from build123d import *

# Parameters (mm, degrees)
CYLINDER003_R               = 0.62
CYLINDER003_DEPTH           = 0.5
CYLINDER002_R               = 0.62
CYLINDER002_DEPTH           = 0.5
CYLINDER001_R               = 0.62
CYLINDER001_DEPTH           = 0.5
CYLINDER001_PLACEMENT_ANGLE = -2
CYLINDER_R                  = 80
CYLINDER_DEPTH              = 0.5


with BuildPart() as cilindro003:
    # Cylinder003 → Cylinder003 (new body)
    with BuildSketch(Plane(origin=(0, 72, 0), x_dir=(1, 0, 0), z_dir=(0, 0, 1))):
        Circle(CYLINDER003_R)
    extrude(amount=CYLINDER003_DEPTH)


with BuildPart() as cilindro002:
    # Cylinder002 → Cylinder002 (new body)
    with BuildSketch(Plane(origin=(-72, -7, 0), x_dir=(1, 0, 0), z_dir=(0, 0, 1))):
        Circle(CYLINDER002_R)
    extrude(amount=CYLINDER002_DEPTH)


with BuildPart() as cilindro001:
    # Cylinder001 → Cylinder001 (new body)
    with BuildSketch(Plane.XY):
        Circle(CYLINDER001_R)
    extrude(amount=CYLINDER001_DEPTH)


with BuildPart() as cilindro001_1:
    # Cylinder001 placement: moved
    add(cilindro001.part.moved(Location((72, -7, 0))).rotate(Axis((72, -7, 0), (0, 0, 1)), CYLINDER001_PLACEMENT_ANGLE))


with BuildPart() as cut002:
    # Cylinder → Cylinder (new body)
    with BuildSketch(Plane.XY):
        Circle(CYLINDER_R)
    extrude(amount=CYLINDER_DEPTH)

    # Cut: cut Cilindro001
    add(cilindro001_1.part, mode=Mode.SUBTRACT)

    # Cut001: cut Cilindro002
    add(cilindro002.part, mode=Mode.SUBTRACT)

    # Cut002: cut Cilindro003
    add(cilindro003.part, mode=Mode.SUBTRACT)


with BuildPart() as cut002_1:
    # Cut002 placement: moved
    add(cut002.part.moved(Location((0, 0, -1))))


solid = cut002_1.part
CAD build for the part. Positions are in the model's coordinates, mm. Round coordinates to 2 decimals unless told otherwise and drop trailing zeros. Loops run counter-clockwise (first coordinate to the right, second up) from the corner with the lowest first, then second, coordinate; pieces in that order, holes last.
(1) Cut at A-A (y = -37.5). Give the cut face in (x, z).
(2) Wall check: line 1 along Y through (x, z) = (0, -0.75); line 2 along Y through (x, z) = (72, -0.75); line 3 along X through (y, z) = (3, -0.9). Give the ranges that are in metal, low to high.
(3) Cut at C-C (z = -0.8). Give the cut face in (x, y), plus the area to 3 significant figures.
(4) Cut at B-B (x = 39). Give the cut face in (y, z).
Findings below:
1. outline: (-70.67, -1) - (70.67, -1) - (70.67, -0.5) - (-70.67, -0.5) - close
2. line 1: y = -80 to 71.38, 72.62 to 80
2. line 2: y = -34.87 to -7.62, -6.38 to 34.87
2. line 3: x = -79.94 to 79.94
3. outline: circle Ø160 at (0, 0); hole circle Ø1.24 at (-72, -7); hole circle Ø1.24 at (0, 72); hole circle Ø1.24 at (72, -7)
3. area: 20,100 mm2
4. outline: (-69.85, -1) - (69.85, -1) - (69.85, -0.5) - (-69.85, -0.5) - close
